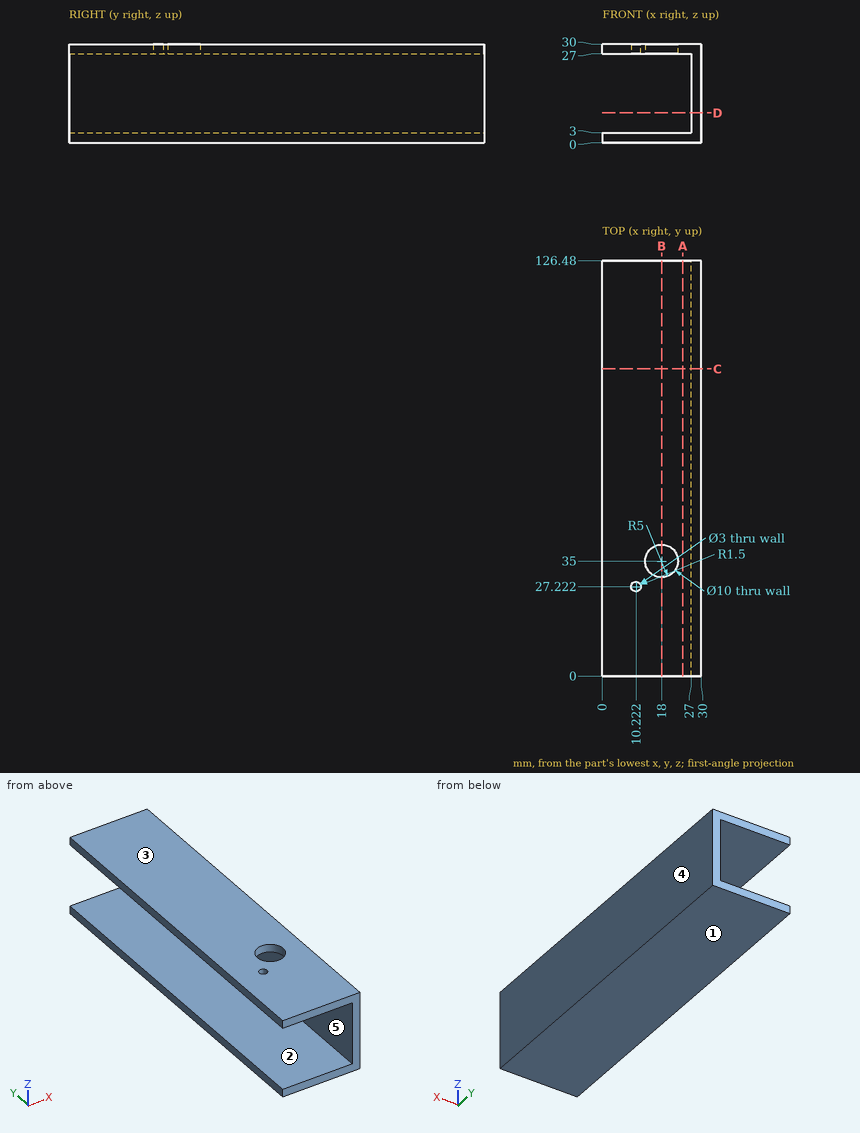
Job drawing, mm, ordinate dimensions from the low corner. One solid piece. A direction names the side the tool comes from. Coordinates: 2 decimals unless noted, no trailing zeros. Order: outer loops, then holes, each group sorted by start corner. A loop starts at its lowest first (then second) coordinate and runs counter-clockwise, first axis right, second up. Notation, with made-up numbers: (36.25, 3) - (45.25, 3) arc R14 cw to (45.25, 22) - close; hole circle Ø8 at (-20.5, 77). An arc over 180 degrees is marked (long way). Use CSV: the item, a comma, the result in double quotes.
Item 1: 3-axis set-ups, long thin cutter, end or side, ignore diameter. For the marked faces 4 and 5: which of +Z, -Z, +X, -X, +Y, -Y reach the whole face in a straight line?
Solved:
face 4,"+Z, -Z, +X, +Y, -Y"
face 5,"-X, +Y, -Y"
Item 2: Mould opens along Z. For the marked faces 1, 2 and 3 say: +Z half, -Z half, draft (parallel to the pull), parting line (faces both ways), or undercut.
Solved:
face 1,"-Z half"
face 2,"undercut"
face 3,"+Z half"
Item 3: Saw through at C-C on y = 93.5. Give the cut face in (x, z).
Solved:
outline,"(0, 0) - (30, 0) - (30, 30) - (0, 30) - (0, 27) - (27, 27) - (27, 3) - (0, 3) - close"
Item 4: Saw through at A-A on x = 24.5. Give the cut face in (y, z), and give its area (3 significant figures).
Solved:
outline,"(0, 0) - (126.48, 0) - (126.48, 3) - (0, 3) - close; (0, 27) - (126.48, 27) - (126.48, 30) - (0, 30) - close"
area,"759 mm²"
Item 5: Drop flat-ended pins along their axis: P1, Ø9, axis at x = 18, y = 35, coming from the +Z side; P2, Ø12, axis at y = 60, z = 16, coming from the -X side. Give the stop position or say it passes through.
Solved:
P1,"stops at z = 3"
P2,"stops at x = 27"
Item 6: Probe probe 1 along Z at (x, y) = (12.5, 114); probe 2 along Y at (x, z) = (18, 28.75); probe 3 along X at (y, z) = (15, 25.5). List the from-to ranges inside material, lowest first.
Solved:
probe 1,"z = 0 to 3, 27 to 30"
probe 2,"y = 0 to 30, 40 to 126.48"
probe 3,"x = 27 to 30"
Item 7: Saw through at B-B on x = 18. Give the cut face in (y, z).
Solved:
outline,"(0, 0) - (126.48, 0) - (126.48, 3) - (0, 3) - close; (0, 27) - (30, 27) - (30, 30) - (0, 30) - close; (40, 27) - (126.48, 27) - (126.48, 30) - (40, 30) - close"
Item 8: Saw through at D-D on z = 9. Give the cut face in (x, y).
Solved:
outline,"(27, 0) - (30, 0) - (30, 126.48) - (27, 126.48) - close"
